Could you check a few things on this model? Use its own coordinates, in mm. A direction names the side the tool comes from. Give positions to 0.01 mm unless a question says otherwise; leave off trailing zeros. Loops run counter-clockwise (first coordinate to the right, second up) from the corner with the lowest first, then second, coordinate; pieces in that order, holes last. Notation, with made-up numbers: (-13, 64) -> (2, 64) arc R23 ccw to (2, 77) -> close; hole circle Ø10 at (-28, 39). An arc over 180 degrees is marked (long way). Put each result on its own line as item: value.
```python
from build123d import *

# Parameters (mm, degrees)
F0_R      = 17.5
F1_DEPTH  = 25
F2_R      = 16.25
F3_DEPTH  = 25
F4_R      = 14
F5_DEPTH  = 50
F6_R      = 13.05
F7_DEPTH  = 25
F8_R      = 12
F9_DEPTH  = 25
F10_R     = 10.925
F11_DEPTH = 25
F12_SIZE  = 2


with BuildPart() as f1:
    # F0 (on Front) → F1 (new body)
    with BuildSketch(Plane.XZ):
        Circle(F0_R)
    extrude(amount=F1_DEPTH)

    # F2 (on face) → F3 (join)
    with BuildSketch(Plane(origin=(0, 0, 0), x_dir=(-1, 0, 0), z_dir=(0, 1, 0))):
        Circle(F2_R)
    extrude(amount=F3_DEPTH)

    # F4 (on face) → F5 (join)
    with BuildSketch(Plane(origin=(0, 25, 0), x_dir=(-1, 0, 0), z_dir=(0, 1, 0))):
        Circle(F4_R)
    extrude(amount=F5_DEPTH)

    # F6 (on face) → F7 (join)
    with BuildSketch(Plane(origin=(0, 75, 0), x_dir=(-1, 0, 0), z_dir=(0, 1, 0))):
        Circle(F6_R)
    extrude(amount=F7_DEPTH)

    # F8 (on face) → F9 (join)
    with BuildSketch(Plane(origin=(0, 100, 0), x_dir=(-1, 0, 0), z_dir=(0, 1, 0))):
        Circle(F8_R)
    extrude(amount=F9_DEPTH)

    # F10 (on face) → F11 (join)
    with BuildSketch(Plane(origin=(0, 125, 0), x_dir=(-1, 0, 0), z_dir=(0, 1, 0))):
        Circle(F10_R)
    extrude(amount=F11_DEPTH)

    # F12
    f12_edges = [f1.edges().sort_by_distance(p)[0] for p in [
        (10.925, 150, 0),
    ]]
    chamfer(f12_edges, length=F12_SIZE)


solid = f1.part
```
1. If we section it at B-B (z = 0): List the corners of the cut face in (x, y) for me (3 decimals), then the cut area to 3 significant figures.
Recorded:
outline: (-17.5, -25) -> (17.5, -25) -> (17.5, 0) -> (16.25, 0) -> (16.25, 25) -> (14, 25) -> (14, 75) -> (13.05, 75) -> (13.05, 100) -> (12, 100) -> (12, 125) -> (10.925, 125) -> (10.925, 148) -> (8.925, 150) -> (-8.925, 150) -> (-10.925, 148) -> (-10.925, 125) -> (-12, 125) -> (-12, 100) -> (-13.05, 100) -> (-13.05, 75) -> (-14, 75) -> (-14, 25) -> (-16.25, 25) -> (-16.25, 0) -> (-17.5, 0) -> close
area: 4,880 mm^2
2. If we section it at A-A (x = 0): List the corners of the cut face in (y, z) for me (3 decimals), then the cut area to 3 significant figures.
Recorded:
outline: (-25, -17.5) -> (0, -17.5) -> (0, -16.25) -> (25, -16.25) -> (25, -14) -> (75, -14) -> (75, -13.05) -> (100, -13.05) -> (100, -12) -> (125, -12) -> (125, -10.925) -> (148, -10.925) -> (150, -8.925) -> (150, 8.925) -> (148, 10.925) -> (125, 10.925) -> (125, 12) -> (100, 12) -> (100, 13.05) -> (75, 13.05) -> (75, 14) -> (25, 14) -> (25, 16.25) -> (0, 16.25) -> (0, 17.5) -> (-25, 17.5) -> close
area: 4,880 mm^2
3. I'm going to push flat-ended pins straight in: pin 1 (12 mm diameter, centred on x = -14, z = -7, fed in from +Y); pin 2 (1 mm diameter, centred on x = -11.5, z = 0, fed in from +Y); pin 3 (3 mm diameter, centred on y = 54.5, z = 5.5, fed in from -X). Where does each tip first touch, or does it pass through?
Recorded:
pin 1: stops at y = 149.27
pin 2: stops at y = 125
pin 3: stops at x = -13.42
4. For faces 3 (the face through (0, -25, 0)), 4 (the face through (9.62, 87.32, 8.82)), which set-ups out of +Z, -Z, +X, -X, +Y, -Y let a thin tool reach every point of the face, with its end or its side?
Recorded:
face 3: +Z, -Z, +X, -X, -Y
face 4: +Y
5. I need wall thicknesses on line 1 (Y direction, x = 4, z = 15.5); line 2 (X direction, y = 116.5, z = -8); line 3 (Y direction, x = 9.5, z = -14). Which ranges of each line are inside material? Lowest first, please.
Recorded:
line 1: y = -25 to 25
line 2: x = -8.94 to 8.94
line 3: y = -25 to 0
6. Thinking about a two-plate mould opening in Z: for faces 1 (the face through (13.3, 25, 4.9)), 2 (the face through (-15.5, 12.32, 4.88)), which applies, pulls with the +Z half, pulls with the -Z half, needs draft (parallel to the pull), parting line crosses it, or undercut?
Recorded:
face 1: needs draft
face 2: parting line crosses it
7. If we section it at D-D (y = 111): List the corners of the cut face in (x, z) for me.
Recorded:
outline: circle Ø24 at (0, 0)
8. If we section it at C-C (y = -12): List the corners of the cut face in (x, z) for me.
Recorded:
outline: circle Ø35 at (0, 0)
